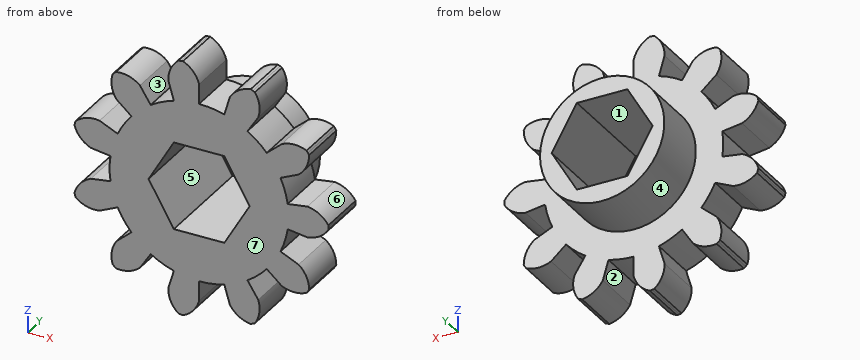
```python
from build123d import *

# Parameters (mm, degrees)
F1_DEPTH = 6.35
F2_R     = 7.9375
F3_DEPTH = 7.366
F5_DEPTH = 25.4
F6_DEPTH = 25.4


with BuildPart() as f1:
    # F0 (on Front) → F1 (new body)
    with BuildSketch(Plane.XZ):
        with BuildLine():
            Line((-3.934953, 13.404367), (-3.219507, 10.967209))
            ThreePointArc((-3.219507, 10.967209), (-4.747864, 10.397244), (-6.179525, 9.615528))
            Line((-6.179525, 9.615528), (-7.552752, 11.752312))
            ThreePointArc((-7.552752, 11.752312), (-8.964411, 12.560176), (-10.587279, 12.66845))
            Line((-10.587279, 12.66845), (-10.813072, 12.47975))
            Line((-10.813072, 12.47975), (-11.031997, 12.283124))
            ThreePointArc((-11.031997, 12.283124), (-11.155886, 10.661374), (-10.557241, 9.149075))
            Line((-10.557241, 9.149075), (-8.637743, 7.485606))
            ThreePointArc((-8.637743, 7.485606), (-9.615332, 6.17983), (-10.397094, 4.748194))
            Line((-10.397094, 4.748194), (-12.707559, 5.803348))
            ThreePointArc((-12.707559, 5.803348), (-14.331886, 5.719766), (-15.755667, 4.933463))
            Line((-15.755667, 4.933463), (-15.843597, 4.652646))
            Line((-15.843597, 4.652646), (-15.921465, 4.368874))
            ThreePointArc((-15.921465, 4.368874), (-15.148902, 2.937591), (-13.827679, 1.989016))
            Line((-13.827679, 1.989016), (-11.313556, 1.627377))
            ThreePointArc((-11.313556, 1.627377), (-11.43, 0.000363), (-11.313659, -1.626659))
            Line((-11.313659, -1.626659), (-13.827806, -1.988138))
            ThreePointArc((-13.827806, -1.988138), (-15.149089, -2.936629), (-15.921742, -4.367864))
            Line((-15.921742, -4.367864), (-15.843893, -4.65164))
            Line((-15.843893, -4.65164), (-15.75598, -4.932463))
            ThreePointArc((-15.75598, -4.932463), (-14.332249, -5.718857), (-12.707927, -5.802541))
            Line((-12.707927, -5.802541), (-10.397395, -4.747534))
            ThreePointArc((-10.397395, -4.747534), (-9.615724, -6.179219), (-8.638218, -7.485058))
            Line((-8.638218, -7.485058), (-10.557822, -9.148404))
            ThreePointArc((-10.557822, -9.148404), (-11.156563, -10.660665), (-11.032776, -12.282424))
            Line((-11.032776, -12.282424), (-10.813864, -12.479064))
            Line((-10.813864, -12.479064), (-10.588083, -12.667778))
            ThreePointArc((-10.588083, -12.667778), (-8.965208, -12.559607), (-7.553498, -11.751832))
            Line((-7.553498, -11.751832), (-6.180135, -9.615136))
            ThreePointArc((-6.180135, -9.615136), (-4.748524, -10.396943), (-3.220203, -10.967005))
            Line((-3.220203, -10.967005), (-3.935804, -13.404117))
            ThreePointArc((-3.935804, -13.404117), (-3.621907, -15.000016), (-2.640982, -16.297402))
            Line((-2.640982, -16.297402), (-2.35051, -16.344473))
            Line((-2.35051, -16.344473), (-2.058545, -16.381163))
            ThreePointArc((-2.058545, -16.381163), (-0.751777, -15.412771), (-0.000887, -13.97))
            Line((-0.000887, -13.97), (-0.000725, -11.43))
            ThreePointArc((-0.000725, -11.43), (1.6263, -11.313711), (3.220203, -10.967005))
            Line((3.220203, -10.967005), (3.935804, -13.404117))
            ThreePointArc((3.935804, -13.404117), (5.062679, -14.576967), (6.589305, -15.13807))
            Line((6.589305, -15.13807), (6.859114, -15.020627))
            Line((6.859114, -15.020627), (7.124567, -14.893644))
            ThreePointArc((7.124567, -14.893644), (7.700339, -13.372489), (7.552006, -11.752791))
            Line((7.552006, -11.752791), (6.178914, -9.61592))
            ThreePointArc((6.178914, -9.61592), (7.484784, -8.638455), (8.638218, -7.485058))
            Line((8.638218, -7.485058), (10.557822, -9.148404))
            ThreePointArc((10.557822, -9.148404), (12.1399, -9.525834), (13.727535, -9.172507))
            Line((13.727535, -9.172507), (13.891018, -8.927838))
            Line((13.891018, -8.927838), (14.045679, -8.677499))
            ThreePointArc((14.045679, -8.677499), (13.707651, -7.086537), (12.707191, -5.804154))
            Line((12.707191, -5.804154), (10.396792, -4.748853))
            ThreePointArc((10.396792, -4.748853), (10.966902, -3.220551), (11.313659, -1.626659))
            Line((11.313659, -1.626659), (13.827806, -1.988138))
            ThreePointArc((13.827806, -1.988138), (15.362788, -1.450316), (16.507369, -0.294739))
            Line((16.507369, -0.294739), (16.512622, -0.000524))
            Line((16.512622, -0.000524), (16.507388, 0.293691))
            ThreePointArc((16.507388, 0.293691), (15.36288, 1.449341), (13.827932, 1.987261))
            Line((13.827932, 1.987261), (11.313762, 1.625941))
            ThreePointArc((11.313762, 1.625941), (10.967107, 3.219855), (10.397094, 4.748194))
            Line((10.397094, 4.748194), (12.707559, 5.803348))
            ThreePointArc((12.707559, 5.803348), (13.7081, 7.085667), (14.04623, 8.676607))
            Line((14.04623, 8.676607), (13.891585, 8.926957))
            Line((13.891585, 8.926957), (13.728117, 9.171636))
            ThreePointArc((13.728117, 9.171636), (12.140504, 9.525064), (10.558402, 9.147734))
            Line((10.558402, 9.147734), (8.638693, 7.48451))
            ThreePointArc((8.638693, 7.48451), (7.485332, 8.63798), (6.179525, 9.615528))
            Line((6.179525, 9.615528), (7.552752, 11.752312))
            ThreePointArc((7.552752, 11.752312), (7.701187, 13.372001), (7.125513, 14.893192))
            Line((7.125513, 14.893192), (6.860068, 15.020192))
            Line((6.860068, 15.020192), (6.590266, 15.137652))
            ThreePointArc((6.590266, 15.137652), (5.063604, 14.576646), (3.936655, 13.403867))
            Line((3.936655, 13.403867), (3.220899, 10.9668))
            ThreePointArc((3.220899, 10.9668), (1.627018, 11.313607), (0, 11.43))
            Line((0, 11.43), (0, 13.97))
            ThreePointArc((0, 13.97), (-0.750798, 15.412819), (-2.057505, 16.381293))
            Line((-2.057505, 16.381293), (-2.349472, 16.344622))
            Line((-2.349472, 16.344622), (-2.639948, 16.29757))
            ThreePointArc((-2.639948, 16.29757), (-3.620955, 15.000246), (-3.934953, 13.404367))
        make_face()
    extrude(amount=F1_DEPTH)

    # F2 (on Front) → F3 (join)
    with BuildSketch(Plane.XZ):
        Circle(F2_R)
    extrude(amount=-F3_DEPTH)

    # F4 (on Front) → F5 (cut)
    with BuildSketch(Plane.XZ):
        Polygon((3.226233, -5.588), (6.452467, 0), (3.226233, 5.588), (-3.226233, 5.588), (-6.452467, 0), (-3.226233, -5.588), align=None)
    extrude(amount=-F5_DEPTH, mode=Mode.SUBTRACT)

    # F5_face (on face) → F6 (cut)
    with BuildSketch(Plane(origin=(0, 0, 0), x_dir=(1, 0, 0), z_dir=(0, 1, 0))):
        Polygon((6.452467, 0), (3.226233, 5.588), (-3.226233, 5.588), (-6.452467, 0), (-3.226233, -5.588), (3.226233, -5.588), align=None)
    extrude(amount=-F6_DEPTH, mode=Mode.SUBTRACT)


solid = f1.part
```
CAD build for the part. Positions are in the model's coordinates, mm. Face numbers are marked on the shaded views. A direction names the side the tool comes from. Round coordinates to 2 decimals unless told otherwise and drop trailing zeros. Order: outer loops, then holes, each group sorted by start corner. A loop starts at its lowest first (then second) coordinate and runs counter-clockwise, first axis right, second up.
Q1. Drop flat-ended pins along their axis: pin 1 (6 mm diameter, centred on y = 2.5, z = 2, fed in from -X); pin 2 (1.5 mm diameter, centred on y = -1, z = -4.5, fed in from +X); pin 3 (6 mm diameter, centred on x = 8, y = -5, fed in from -Z); pin 4 (3 mm diameter, centred on y = 2, z = 9.5, fed in from +X). Give the stop position or say it passes through.
Q2. Slice it at B-B (x = -0.5). Write the cut outline in (y, z).
Q3. Two-plate mould, pull along X, no slides. Class the marked faces 5, 6 and 7: pulls with the +X half, pulls with the -X half, needs draft (parallel to the pull), parting line crosses it, or undercut.
Q4. Which spindle directions (+Z, -Z, +X, -X, +Y, -Y) get a long thin tool onto all of the face, cutting with end or side? Do the marked faces 1, 2, 3 and 4. Say none if no direction does.
Q5. Slice it at C-C (z = -2.5). Write the cut outline in (x, y).
Q6. Wall check: L1, parallel to Y at x = -11, z = -2; L2, parallel to X at y = -3.75, z = -14; L3, parallel to Z at x = -2.5, y = 2. Give the ranges that are in metal, low to high.
Q7. Slice it at A-A (y = 1). Write the cut outline in (x, z) (1 decimal).
Q8. Slice it at D-D (x = -7). Write the cut outline in (y, z).
Results below:
1. pin 1: stops at x = -15.64
1. pin 2: stops at x = 11.49
1. pin 3: stops at z = -15.14
1. pin 4: passes through
2. outline: (-6.35, -15.08) - (0, -15.08) - (0, -7.92) - (7.37, -7.92) - (7.37, -5.59) - (-6.35, -5.59) - close; (-6.35, 5.59) - (7.37, 5.59) - (7.37, 7.92) - (0, 7.92) - (0, 15.08) - (-6.35, 15.08) - close
3. face 5: undercut
3. face 6: pulls with the +X half
3. face 7: needs draft
4. face 1: +Y, -Y
4. face 2: -Z, +Y, -Y
4. face 3: +Z, +Y, -Y
4. face 4: +Y
5. outline: (-14.69, -6.35) - (-5.01, -6.35) - (-5.01, 7.37) - (-7.53, 7.37) - (-7.53, 0) - (-14.69, 0) - close; (5.01, -6.35) - (11.15, -6.35) - (11.15, 0) - (7.53, 0) - (7.53, 7.37) - (5.01, 7.37) - close
6. L1: y = -6.35 to 0
6. L2: x = -3.91 to -0.01, 4.38 to 7.56
6. L3: z = -7.53 to -5.59, 5.59 to 7.53
7. outline: circle Ø15.9 at (0, 0); hole (-6.5, 0) - (-3.2, -5.6) - (3.2, -5.6) - (6.5, 0) - (3.2, 5.6) - (-3.2, 5.6) - close
8. outline: (-6.35, -10.89) - (0, -10.89) - (0, -3.74) - (7.37, -3.74) - (7.37, 3.74) - (0, 3.74) - (0, 10.89) - (-6.35, 10.89) - close
